```python
from build123d import *

# Parameters (mm, degrees)
F1_DEPTH = 109.8860576749
F2_T     = -2.54
F3_R     = 5.08
F4_R     = 5.08


with BuildPart() as f1:
    # F0 (on Top) → F1 (new body)
    with BuildSketch(Plane.XY):
        Polygon((84.8518013954, -59.6191361547), (84.8518013954, 69.0497234464), (0.4590898752, 69.0497234464), (-54.9942553043, 22.0465362072), (-54.9942553043, -21.6257423162), (-3.1802803278, -53.0151873827), (52.0924478769, -39.3676012754), (62.5555962324, -52.7877360582), (65.0224879491, -59.6191361547), align=None)
    extrude(amount=F1_DEPTH)

    # F2
    f2_openings = [f1.faces().sort_by_distance(p)[0] for p in [
        (22.309592, 7.913715, 109.886058),
    ]]
    offset(amount=F2_T, openings=f2_openings, kind=Kind.INTERSECTION)

    # F3
    f3_edges = [f1.edges().sort_by_distance(p)[0] for p in [
        (74.558802, -57.079136, 2.54),
        (65.806549, -54.311968, 2.54),
        (58.945027, -44.025799, 2.54),
        (25.158494, -43.401678, 2.54),
        (-27.610013, -35.245657, 2.54),
        (-52.454255, 0.337522, 2.54),
        (-25.531758, 43.689762, 2.54),
        (41.85127, 66.509723, 2.54),
        (82.311801, 4.715294, 2.54),
    ]]
    fillet(f3_edges, radius=F3_R)

    # F4
    f4_edges = [f1.edges().sort_by_distance(p)[0] for p in [
        (84.851801, 4.715294, 0),
        (42.655446, 69.049723, 0),
        (-27.267583, 45.54813, 0),
        (-54.994255, 0.210397, 0),
        (-29.087268, -37.320465, 0),
        (24.456084, -46.191394, 0),
        (57.324022, -46.077669, 0),
        (63.789042, -56.203436, 0),
        (74.937145, -59.619136, 0),
    ]]
    fillet(f4_edges, radius=F4_R)


solid = f1.part
```
Part model, mm, in its own coordinate system. A direction names the side the tool comes from. Coordinates: 2 decimals unless noted, no trailing zeros. Order: outer loops, then holes, each group sorted by start corner. A loop starts at its lowest first (then second) coordinate and runs counter-clockwise, first axis right, second up. Notation, with made-up numbers: (10.25, 86) - (55.25, 86) arc R25 cw to (55.25, 101) - close; hole circle Ø1 at (63, 72.25). An arc over 180 degrees is marked (long way). Return JSON: item names as keys, results as strings. Group by question number.
Item 1: Cut at A-A (z = 39). List the corners of the cut face in (x, y).
Item 2: Cut at B-B (x = 74). List the corners of the cut face in (y, z), plus the area to 3 significant figures.
Item 3: Pin check, flat tips, straight feed: pin 1 (8 mm diameter, centred on x = 53.5, z = 93.5, fed in from -Y); pin 2 (3 mm diameter, centred on y = -33.5, z = 76.5, fed in from -X); pin 3 (12 mm diameter, centred on y = 29, z = 49, fed in from -X). Stop position of each tip, or through.
Item 4: Drill centre lines: probe 1 along X at (y, z) = (17, 50); probe 2 along Y at (x, z) = (67, 92); probe 3 along Z at (x, y) = (64, -12.5). Where is each one in solid material? Low to high. Write a range as from..to.
Item 5: Which spindle directions (+Z, -Z, +X, -X, +Y, -Y) get a long thin tool onto all of the face, cutting with end or side? Do faces 5 (the face through (75.076, -58.171, 1.528)), 6 (the face through (41.285, 65.061, 4.068)), 7 (the face through (26.12, -44.29, 1.53)). Say none if no direction does.
Item 6: Cut at C-C (y = 2). List the corners of the cut face in (x, z), plus the area to 3 significant figures.
Item 7: Pull direction Y, two halves, no side cores. Call faces 1 (the face through (-26.51, -34.22, 4.07)), 2 (the face through (80.863, 5.58, 4.068)), 3 (the face through (24.069, -46.287, 56.749)), 4 (the face through (-22, 48, 109.886)): pulls with the +Y half, pulls with the -Y half, needs draft (parallel to the pull), parting line crosses it, or undercut.
Check values:
{
 "1": {"outline": "(-54.99, -21.63) - (-3.18, -53.02) - (52.09, -39.37) - (62.56, -52.79) - (65.02, -59.62) - (84.85, -59.62) - (84.85, 69.05) - (0.46, 69.05) - (-54.99, 22.05) - close; hole (-52.45, -20.19) - (-2.77, -50.3) - (53.08, -36.51) - (64.81, -51.54) - (66.81, -57.08) - (82.31, -57.08) - (82.31, 66.51) - (1.39, 66.51) - (-52.45, 20.87) - close"},
 "2": {"outline": "(-59.62, 5.08) arc R5.08 ccw to (-54.54, 0) - (63.97, 0) arc R5.08 ccw to (69.05, 5.08) - (69.05, 109.89) - (66.51, 109.89) - (66.51, 7.62) arc R5.08 cw to (61.43, 2.54) - (-52, 2.54) arc R5.08 cw to (-57.08, 7.62) - (-57.08, 109.89) - (-59.62, 109.89) - close", "area": "872 mm2"},
 "3": {"pin 1": "stops at y = -46.3", "pin 2": "stops at x = -37.87", "pin 3": "stops at x = -53.87"},
 "4": {"probe 1": "x = -54.99..-52.45, 82.31..84.85", "probe 2": "y = -59.62..-57.08, 66.51..69.05", "probe 3": "z = 0..2.54"},
 "5": {"face 5": "-Z, +X, -X, -Y", "face 6": "+Z", "face 7": "-Z, -Y"},
 "6": {"outline": "(-54.99, 5.08) arc R5.08 ccw to (-49.91, 0) - (79.77, 0) arc R5.08 ccw to (84.85, 5.08) - (84.85, 109.89) - (82.31, 109.89) - (82.31, 7.62) arc R5.08 cw to (77.23, 2.54) - (-47.37, 2.54) arc R5.08 cw to (-52.45, 7.62) - (-52.45, 109.89) - (-54.99, 109.89) - close", "area": "901 mm2"},
 "7": {"face 1": "undercut", "face 2": "undercut", "face 3": "pulls with the -Y half", "face 4": "needs draft"}
}
